Work out the finished part from the listing and answer in its coordinate system (mm). A direction names the side the tool comes from. Give positions to 0.01 mm unless a question says otherwise; leave off trailing zeros. Loops run counter-clockwise (first coordinate to the right, second up) from the corner with the lowest first, then second, coordinate; pieces in that order, holes last. Notation, with made-up numbers: M 51.25,55 L 74.25,55 A16 cw 74.25,68 Z; hole C 21.25,21.5 d10. An arc over 180 degrees is marked long. Use a Markdown table: item, result.
```python
from build123d import *

# Parameters (mm, degrees)
SKETCH_2_R      = 5
EXTRUDE_1_DEPTH = 50
THREAD_1_PITCH  = 1
THREAD_1_HEIGHT = 10
THREAD_1_RADIUS = 5
SKETCH_8_R      = 7.146780715
EXTRUDE_2_DEPTH = 20


with BuildPart() as part:
    # Sketch 2 → Бобышка-Вытянуть1 (new body)
    with BuildSketch(Plane.XY):
        Circle(SKETCH_2_R)
    extrude(amount=EXTRUDE_1_DEPTH)

    # Резьба1: sweep along a helix
    with BuildLine() as thread_1_path:
        Helix(THREAD_1_PITCH, THREAD_1_HEIGHT, THREAD_1_RADIUS, center=(0, 0, 50), direction=(0, 0, -1))
    # Sketch 2 2 → Резьба1 (sweep, cut)
    with BuildSketch(Plane(origin=(-5, 0, 50), x_dir=(-1, 0, 0), z_dir=(0, -1, 0))):
        Polygon((0, 0), (0, 0.874999997), (-0.541265875, 0.562499999), (-0.541265875, 0.312499999), align=None)
    sweep(path=thread_1_path.line, is_frenet=True, mode=Mode.SUBTRACT)

    # Эскиз8 → Бобышка-Вытянуть2 (add)
    with BuildSketch(Plane.XY.offset(50)):
        Circle(SKETCH_8_R)
    extrude(amount=-EXTRUDE_2_DEPTH)


solid = part.part
```
(1) A cutting plane is placed at D-D (z = 21.5). Write down the section's boundary in (x, y).
Entries:
| item | result |
|---|---|
| outline | C 0,0 d10 |
(2) Given P1, Ø3, axis at y = 2, z = 6.5, coming from the +X side; P2, Ø1, axis at y = -4, z = 13, coming from the +X side; P3, Ø5, axis at y = 5.5, z = 21, coming from the +X side, each flat-ended and moving along its own axis, determine where each tip first touches the part or whether it passes through.
Entries:
| item | result |
|---|---|
| P1 | stops at x = 4.97 |
| P2 | stops at x = 3.57 |
| P3 | stops at x = 4 |
(3) Which of the six approach directions +Z, -Z, +X, -X, +Y, -Y give full straight-line access (tool end or side, diameter ignored) to faces 1 (the cylindrical face through (-5.67, -4.35, 40.14)), 2 (the cylindrical face through (-1.08, -4.88, 14.79))?
Entries:
| item | result |
|---|---|
| face 1 | +Z, -Z |
| face 2 | -Z |
(4) Consider probe 1 along Z at (x, y) = (-1, -5.25); probe 2 along Y at (x, z) = (0, 5.5); probe 3 along Y at (x, z) = (0.25, 34). Determine where each line is inside the solid, lowest interval first. Write a range as [from, to].
Entries:
| item | result |
|---|---|
| probe 1 | z = [30, 50] |
| probe 2 | y = [-5, 5] |
| probe 3 | y = [-7.14, 7.14] |
(5) A cutting plane is placed at A-A (x = 0). Write down the section's boundary in (y, z), and give its area (3 significant figures).
Entries:
| item | result |
|---|---|
| outline | M -7.15,30 L -5,30 L -5,0 L 5,0 L 5,30 L 7.15,30 L 7.15,50 L -7.15,50 Z |
| area | 586 mm² |
(6) A cutting plane is placed at C-C (z = 41). Write down the section's boundary in (x, y).
Entries:
| item | result |
|---|---|
| outline | C 0,0 d14.29 |
